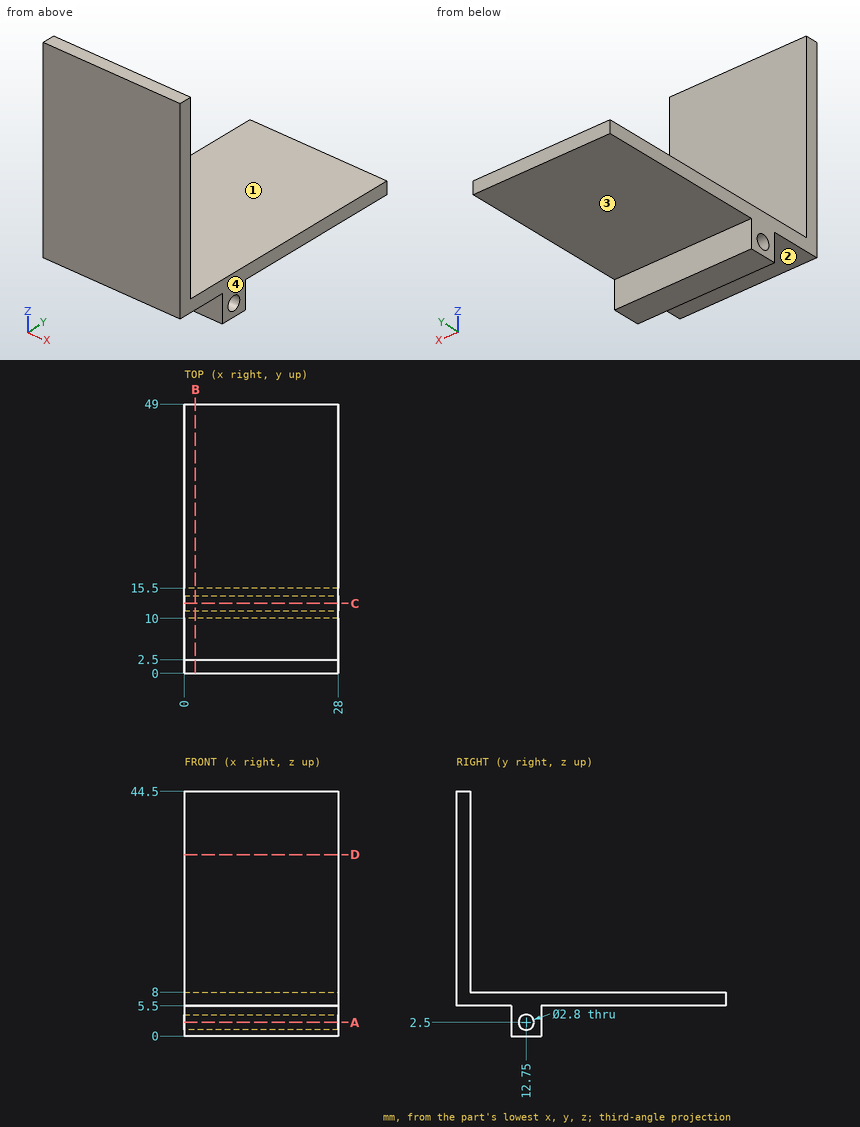
Geometry: see drawing. Coordinates: mm, zero at the bounding-box minimum. A direction names the side the tool comes from. Give positions to 0.01 mm unless a question says otherwise; leave off trailing zeros. Loops run counter-clockwise (first coordinate to the right, second up) from the corner with the lowest first, then second, coordinate; pieces in that order, holes last. Notation, with made-up numbers: (-6.5, 22) - (36.5, 22) arc R15 cw to (36.5, 26) - close; hole circle Ø2 at (21.25, 74.25). An arc over 180 degrees is marked (long way). Use CSV: the item, a comma, the result in double quotes. Start each with the question number.
1. Section D-D (z = 33). Output: boundary loops of the cut face in (x, y), then the cut area to 3 significant figures.
2. Section B-B (x = 2). Output: boundary loops of the cut face in (y, z).
3. Reachability of the marked faces 1, 2, 3 and 4 from +Z, -Z, +X, -X, +Y, -Y: full face, straight path, thin tool, end or side. Return the list, or none.
4. Section A-A (z = 2.5). Output: boundary loops of the cut face in (x, y).
5. Section C-C (y = 12.75). Output: boundary loops of the cut face in (x, z), then the cut area to 3 significant figures.
6. Pin query (flat end, axial travel): pin 1 (6 mm diameter, centred on x = 11.5, y = 36.5, fed in from +Z); pin 2 (2 mm diameter, centred on y = 12.75, z = 2.5, fed in from -X); pin 3 (14 mm diameter, centred on x = 12, y = 31.5, fed in from -Z); pin 4 (1.6 mm diameter, centred on x = 8.5, z = 4, fed in from +Y). Return the tip coordinate at first contact, or that it passes through.
7. Ray query, L1, parallel to Y at x = 7, z = 2.5; L2, parallel to Y at x = 21.75, z = 40; L3, parallel to Z at x = 3.5, y = 23.5. Return the intervals inside material, ascending.
Response:
1,outline,"(0, 0) - (28, 0) - (28, 2.5) - (0, 2.5) - close"
1,area,"70.0 mm²"
2,outline,"(0, 5.5) - (10, 5.5) - (10, 0) - (15.5, 0) - (15.5, 5.5) - (49, 5.5) - (49, 8) - (2.5, 8) - (2.5, 44.5) - (0, 44.5) - close; hole circle Ø2.8 at (12.75, 2.5)"
3,face 1,"+Z, +X, -X, +Y"
3,face 2,"-Z, +X, -X, -Y"
3,face 3,"-Z, +X, -X, +Y"
3,face 4,"+Z, -Z, +X, +Y, -Y"
4,outline,"(0, 10) - (28, 10) - (28, 11.35) - (0, 11.35) - close; (0, 14.15) - (28, 14.15) - (28, 15.5) - (0, 15.5) - close"
5,outline,"(0, 0) - (28, 0) - (28, 1.1) - (0, 1.1) - close; (0, 3.9) - (28, 3.9) - (28, 8) - (0, 8) - close"
5,area,"146 mm²"
6,pin 1,"z = 8"
6,pin 2,"through"
6,pin 3,"z = 5.5"
6,pin 4,"y = 15.5"
7,L1,"10 to 11.35, 14.15 to 15.5"
7,L2,"0 to 2.5"
7,L3,"5.5 to 8"
